```python
from build123d import *

# Parameters (mm, degrees)
BOSS_EXTRUDE1_DEPTH = 2.54
SKETCH2_W           = 1.27
SKETCH2_H           = 0.381
CUT_EXTRUDE1_DEPTH  = 2.54
SKETCH3_W           = 0.635
SKETCH3_H           = 0.635
BOSS_EXTRUDE2_DEPTH = 5.5
CHAMFER1_SIZE       = 0.1905
SKETCH4_W           = 0.635
SKETCH4_H           = 0.635
BOSS_EXTRUDE3_DEPTH = 2.9
CHAMFER2_SIZE       = 0.1905


with BuildPart() as part:
    # Sketch1 → Boss-Extrude1 (new body)
    with BuildSketch(Plane(origin=(0, 0, 0), x_dir=(1, 0, 0), z_dir=(0, 1, 0))):
        Polygon((0.635, 1.27), (1.27, 0.635), (1.27, -0.635), (0.635, -1.27), (-0.635, -1.27), (-1.27, -0.635), (-1.27, 0.635), (-0.635, 1.27), align=None)
    extrude(amount=BOSS_EXTRUDE1_DEPTH)

    # Sketch2 → Cut-Extrude1 (cut)
    with BuildSketch(Plane(origin=(1.27, 0, 0), x_dir=(0, 0, -1), z_dir=(1, 0, 0))):
        with Locations((0, 0.1905)):
            Rectangle(SKETCH2_W, SKETCH2_H)
    extrude(amount=-CUT_EXTRUDE1_DEPTH, mode=Mode.SUBTRACT)

    # Sketch3 → Boss-Extrude2 (add)
    with BuildSketch(Plane(origin=(0, 2.54, 0), x_dir=(1, 0, 0), z_dir=(0, 1, 0))):
        Rectangle(SKETCH3_W, SKETCH3_H)
    extrude(amount=BOSS_EXTRUDE2_DEPTH)

    # Chamfer1
    chamfer1_edges = [part.edges().sort_by_distance(p)[0] for p in [
        (0.3175, 8.04, 0),
        (0, 8.04, -0.3175),
        (-0.3175, 8.04, 0),
        (0, 8.04, 0.3175),
    ]]
    chamfer(chamfer1_edges, length=CHAMFER1_SIZE)

    # Sketch4 → Boss-Extrude3 (add)
    with BuildSketch(Plane.XZ.offset(-0.381)):
        Rectangle(SKETCH4_W, SKETCH4_H)
    extrude(amount=BOSS_EXTRUDE3_DEPTH)

    # Chamfer2
    chamfer2_edges = [part.edges().sort_by_distance(p)[0] for p in [
        (0.3175, -2.519, 0),
        (0, -2.519, 0.3175),
        (-0.3175, -2.519, 0),
        (0, -2.519, -0.3175),
    ]]
    chamfer(chamfer2_edges, length=CHAMFER2_SIZE)


solid = part.part
```
Part model, mm, in its own coordinate system. Round coordinates to 2 decimals unless told otherwise and drop trailing zeros. Order: outer loops, then holes, each group sorted by start corner. A loop starts at its lowest first (then second) coordinate and runs counter-clockwise, first axis right, second up. Notation, with made-up numbers: M 73,73 L 116,73 A24 cw 116,105 Z; hole C 51.25,-15.75 d3. An arc over 180 degrees is marked long. Answer in a Markdown table with one row per item. Add a question column.
Q1. Cut at C-C on z = -0.45. Give the cut face in (x, y), and give its area (3 significant figures).
Q2. Wall check: L1, parallel to Y at x = 0.3, z = -0.45; L2, parallel to Y at x = -0.6, z = -0.8; L3, parallel to X at y = 4.5, z = 0.25. Give the ranges that are in metal, low to high. Write a range as from..to.
Q3. Cut at D-D on y = 4.25. Give the cut face in (x, z).
Q4. Cut at A-A on y = 1. Give the cut face in (x, z) (3 decimals), and give its area (3 significant figures).
Q5. Cut at B-B on x = 0.5. Give the cut face in (y, z) (3 decimals).
Q6. Pin check, flat tips, straight feed: pin 1 (0.5 mm diameter, centred on y = 6.5, z = 0, fed in from +X); pin 2 (1 mm diameter, centred on x = -0.5, y = 3.5, fed in from +Z); pin 3 (0.7 mm diameter, centred on x = 0, z = 1, fed in from -Y). Stop position of each tip, or through.
Established:
| question | item | result |
|---|---|---|
| 1 | outline | M -1.27,0.38 L 1.27,0.38 L 1.27,2.54 L -1.27,2.54 Z |
| 1 | area | 5.48 mm2 |
| 2 | L1 | y = 0.38..2.54 |
| 2 | L2 | y = 0..2.54 |
| 2 | L3 | x = -0.32..0.32 |
| 3 | outline | M -0.32,-0.32 L 0.32,-0.32 L 0.32,0.32 L -0.32,0.32 Z |
| 4 | outline | M -1.27,-0.635 L -0.635,-1.27 L 0.635,-1.27 L 1.27,-0.635 L 1.27,0.635 L 0.635,1.27 L -0.635,1.27 L -1.27,0.635 Z |
| 4 | area | 5.65 mm2 |
| 5 | outline | M 0,-1.27 L 2.54,-1.27 L 2.54,1.27 L 0,1.27 L 0,0.635 L 0.381,0.635 L 0.381,-0.635 L 0,-0.635 Z |
| 6 | pin 1 | stops at x = 0.32 |
| 6 | pin 2 | stops at z = 0.32 |
| 6 | pin 3 | stops at y = 0 |
